from build123d import *

# Parameters (mm, degrees)
RESSALTO_EXTRUS_O1_DEPTH = 22.7
ESBO_O2_W                = 8.5
ESBO_O2_H                = 3.7
CORTE_EXTRUS_O1_DEPTH    = 9.5
ESBO_O3_W                = 8.527883753
ESBO_O3_H                = 4.058843418
CORTE_EXTRUS_O2_DEPTH    = 9.5
FILETE4_R                = 1


with BuildPart() as part:
    # Esboço1 → Ressalto-extrusão1 (new body)
    with BuildSketch(Plane.XY):
        Polygon((-52.043977441, 13.555253824), (-52.043977441, -1.544746176), (-6.943977441, -1.544746176), (-6.943977441, 25.555253824), (1.556022559, 25.555253824), (1.556022559, 29.255253824), (-6.943977441, 29.255253824), (-6.943977441, 40.455253824), (-20.743977441, 40.455253824), (-20.743977441, 13.555253824), align=None)
    extrude(amount=RESSALTO_EXTRUS_O1_DEPTH)

    # Esboço2 → Corte-extrusão1 (cut)
    with BuildSketch(Plane.XY.offset(22.7)):
        with Locations((-2.693977441, 27.405253824)):
            Rectangle(ESBO_O2_W, ESBO_O2_H)
    extrude(amount=-CORTE_EXTRUS_O1_DEPTH, mode=Mode.SUBTRACT)

    # Esboço3 → Corte-extrusão2 (cut)
    with BuildSketch(Plane(origin=(0, 0, 0), x_dir=(-1, 0, 0), z_dir=(0, 0, -1))):
        with Locations((2.680035565, 27.225832115)):
            Rectangle(ESBO_O3_W, ESBO_O3_H)
    extrude(amount=-CORTE_EXTRUS_O2_DEPTH, mode=Mode.SUBTRACT)

    # Filete4
    filete4_edges = [part.edges().sort_by_distance(p)[0] for p in [
        (-2.693977441, 29.255253824, 13.2),
        (-2.693977441, 25.555253824, 13.2),
        (-2.693977441, 25.555253824, 9.5),
        (-2.693977441, 29.255253824, 9.5),
    ]]
    fillet(filete4_edges, radius=FILETE4_R)


solid = part.part
Part model, mm, in its own coordinate system. A direction names the side the tool comes from. Coordinates: 2 decimals unless noted, no trailing zeros. Loops run counter-clockwise (first coordinate to the right, second up) from the corner with the lowest first, then second, coordinate; pieces in that order, holes last. Notation, with made-up numbers: (-11, -24.75) -> (18, -24.75) arc R28 cw to (18, 5.25) -> close; hole circle Ø3 at (-21.75, 34.25). An arc over 180 degrees is marked (long way). Use a Markdown table: item, result. Add a question column.
Item 1: Band-saw the part on C-C on y = 30. Write the cut outline in (x, z), plus the area to 3 significant figures.
Item 2: Band-saw the part on B-B on x = -33.5. Write the cut outline in (y, z), plus the area to 3 significant figures.
Item 3: Band-saw the part on A-A on z = 5.5. Write the cut outline in (x, y).
Item 4: Which spindle directions (+Z, -Z, +X, -X, +Y, -Y) get a long thin tool onto all of the face, cutting with end or side? Do faces 1 (the flat face through (-20.744, 27, 11)), 2 (the flat face through (-3, 29.255, 11)), 3 (the flat face through (-3, 27, 9.5)), 4 (the flat face through (-3, 27, 13.2)). Say none if no direction does.
Item 5: Flat gauge pins, fed straight in: P1, Ø1.5, axis at x = -4.5, z = 14, coming from the +Y side; P2, Ø0.8, axis at x = -1, y = 27.5, coming from the -Z side; P3, Ø0.8, axis at x = -1.5, z = 11.5, coming from the +Y side; P4, Ø11.5, axis at y = 15, z = 15, coming from the +X side. Where does each tip first touch, or does it go through?
Item 6: Probe probe 1 along Y at (x, z) = (-36, 17.5); probe 2 along X at (y, z) = (7.5, 15); probe 3 along X at (y, z) = (38.5, 1.25). List the from-to ranges inside material, lowest first.
Geometry says:
| question | item | result |
|---|---|---|
| 1 | outline | (-20.74, 0) -> (-6.94, 0) -> (-6.94, 22.7) -> (-20.74, 22.7) -> close |
| 1 | area | 313 mm² |
| 2 | outline | (-1.54, 0) -> (13.56, 0) -> (13.56, 22.7) -> (-1.54, 22.7) -> close |
| 2 | area | 343 mm² |
| 3 | outline | (-52.04, -1.54) -> (-6.94, -1.54) -> (-6.94, 40.46) -> (-20.74, 40.46) -> (-20.74, 13.56) -> (-52.04, 13.56) -> close |
| 4 | face 1 | +Z, -Z, -X, +Y |
| 4 | face 2 | +Z, -Z, +X, +Y |
| 4 | face 3 | -Z, +X, +Y, -Y |
| 4 | face 4 | +Z, +X, +Y, -Y |
| 5 | P1 | through |
| 5 | P2 | z = 9.5 |
| 5 | P3 | y = 29.26 |
| 5 | P4 | x = -6.94 |
| 6 | probe 1 | -1.54 to 13.56 |
| 6 | probe 2 | -52.04 to -6.94 |
| 6 | probe 3 | -20.74 to -6.94 |
